Check sheet for the modelled part. Datum: model origin and axes. Units: mm. Round coordinates to 2 decimals unless told otherwise and drop trailing zeros. Write each loop counter-clockwise with the first axis right and the second up, starting at its lowest first coordinate (ties: lowest second). Pieces come first, ordered by that corner, then holes. Notation, with made-up numbers: (2.5, -28) - (8.5, -28) arc R34 cw to (8.5, 11) - close; hole circle Ø5 at (68, 20). An arc over 180 degrees is marked (long way). Answer as a JSON object with one key per item and string values. Group by question number.
Item 1: Sectioned sample at A-A on x = 90.5. Record the boundary of the cut face in (y, z) (3 decimals), plus the area to 3 significant figures.
Item 2: Thickness scan on line 1 (Y direction, x = 118.11, z = 1) (3 decimals); line 2 (Y direction, x = -101.6, z = 0.75); line 3 (Y direction, x = 139, z = 2.95). Record the ranges inside material, lowest first.
Item 3: Gauge pin test, flat ends, axial feed: P1, Ø5, axis at x = 139.7, y = 0, coming from the -Z side; P2, Ø8, axis at x = -101.6, y = 97.79, coming from the +Z side (3 decimals). Record the tip position at first contact, or that the pin passes through.
Item 4: Sectioned sample at B-B on z = 1.45. Count the separate pieces of the cut face and the enclosed holes in it, plus the area to 3 significant figures.
```python
from build123d import *

# Parameters (mm, degrees)
SKETCH1_W           = 304.8
SKETCH1_H           = 304.8
SKETCH1_R           = 2.54
SKETCH1_R_2         = 3.2639
BOSS_EXTRUDE1_DEPTH = 3.175


with BuildPart() as part:
    # Sketch1 → Boss-Extrude1 (new body)
    with BuildSketch(Plane.XY):
        Rectangle(SKETCH1_W, SKETCH1_H)
        with Locations((-50.8, 127)):
            Circle(SKETCH1_R, mode=Mode.SUBTRACT)
        with Locations((0, 127)):
            Circle(SKETCH1_R, mode=Mode.SUBTRACT)
        with Locations((50.8, 127)):
            Circle(SKETCH1_R, mode=Mode.SUBTRACT)
        with Locations((50.8, -127)):
            Circle(SKETCH1_R, mode=Mode.SUBTRACT)
        with Locations((0, -127)):
            Circle(SKETCH1_R, mode=Mode.SUBTRACT)
        with Locations((-50.8, -127)):
            Circle(SKETCH1_R, mode=Mode.SUBTRACT)
        with Locations((-101.6, 97.79)):
            Circle(SKETCH1_R, mode=Mode.SUBTRACT)
        with Locations((0, 97.79)):
            Circle(SKETCH1_R, mode=Mode.SUBTRACT)
        with Locations((101.6, 97.79)):
            Circle(SKETCH1_R, mode=Mode.SUBTRACT)
        with Locations((101.6, 127)):
            Circle(SKETCH1_R, mode=Mode.SUBTRACT)
        with Locations((-101.6, 127)):
            Circle(SKETCH1_R, mode=Mode.SUBTRACT)
        with Locations((-118.11, 33.02)):
            Circle(SKETCH1_R, mode=Mode.SUBTRACT)
        with Locations((-101.6, -127)):
            Circle(SKETCH1_R, mode=Mode.SUBTRACT)
        with Locations((101.6, -127)):
            Circle(SKETCH1_R, mode=Mode.SUBTRACT)
        with Locations((101.6, -97.79)):
            Circle(SKETCH1_R, mode=Mode.SUBTRACT)
        with Locations((0, -97.79)):
            Circle(SKETCH1_R, mode=Mode.SUBTRACT)
        with Locations((-101.6, -97.79)):
            Circle(SKETCH1_R, mode=Mode.SUBTRACT)
        with Locations((-118.11, -33.02)):
            Circle(SKETCH1_R, mode=Mode.SUBTRACT)
        with Locations((-139.7, 139.7)):
            Circle(SKETCH1_R_2, mode=Mode.SUBTRACT)
        with Locations((-139.7, 0)):
            Circle(SKETCH1_R_2, mode=Mode.SUBTRACT)
        with Locations((-139.7, -139.7)):
            Circle(SKETCH1_R_2, mode=Mode.SUBTRACT)
        with Locations((139.7, -139.7)):
            Circle(SKETCH1_R_2, mode=Mode.SUBTRACT)
        with Locations((139.7, 0)):
            Circle(SKETCH1_R_2, mode=Mode.SUBTRACT)
        with Locations((139.7, 139.7)):
            Circle(SKETCH1_R_2, mode=Mode.SUBTRACT)
        with Locations((118.11, -33.02)):
            Circle(SKETCH1_R, mode=Mode.SUBTRACT)
        with Locations((118.11, 33.02)):
            Circle(SKETCH1_R, mode=Mode.SUBTRACT)
        with BuildLine():
            Line((-101.6, 78.74), (101.6, 78.74))
            ThreePointArc((101.6, 78.74), (106.090128061, 76.880128061), (107.95, 72.39))
            Line((107.95, 72.39), (107.95, 24.765))
            ThreePointArc((107.95, 24.765), (108.693948776, 22.968948776), (110.49, 22.225))
            Line((110.49, 22.225), (120.65, 22.225))
            ThreePointArc((120.65, 22.225), (125.140128061, 20.365128061), (127, 15.875))
            Line((127, 15.875), (127, -15.875))
            ThreePointArc((127, -15.875), (125.140128061, -20.365128061), (120.65, -22.225))
            Line((120.65, -22.225), (110.49, -22.225))
            ThreePointArc((110.49, -22.225), (108.693948776, -22.968948776), (107.95, -24.765))
            Line((107.95, -24.765), (107.95, -72.39))
            ThreePointArc((107.95, -72.39), (106.090128061, -76.880128061), (101.6, -78.74))
            Line((101.6, -78.74), (-101.6, -78.74))
            ThreePointArc((-101.6, -78.74), (-106.090128061, -76.880128061), (-107.95, -72.39))
            Line((-107.95, -72.39), (-107.95, -24.765))
            ThreePointArc((-107.95, -24.765), (-108.693948776, -22.968948776), (-110.49, -22.225))
            Line((-110.49, -22.225), (-120.65, -22.225))
            ThreePointArc((-120.65, -22.225), (-125.140128061, -20.365128061), (-127, -15.875))
            Line((-127, -15.875), (-127, 15.875))
            ThreePointArc((-127, 15.875), (-125.140128061, 20.365128061), (-120.65, 22.225))
            Line((-120.65, 22.225), (-110.49, 22.225))
            ThreePointArc((-110.49, 22.225), (-108.693948776, 22.968948776), (-107.95, 24.765))
            Line((-107.95, 24.765), (-107.95, 72.39))
            ThreePointArc((-107.95, 72.39), (-106.090128061, 76.880128061), (-101.6, 78.74))
        make_face(mode=Mode.SUBTRACT)
    extrude(amount=BOSS_EXTRUDE1_DEPTH)


solid = part.part
```
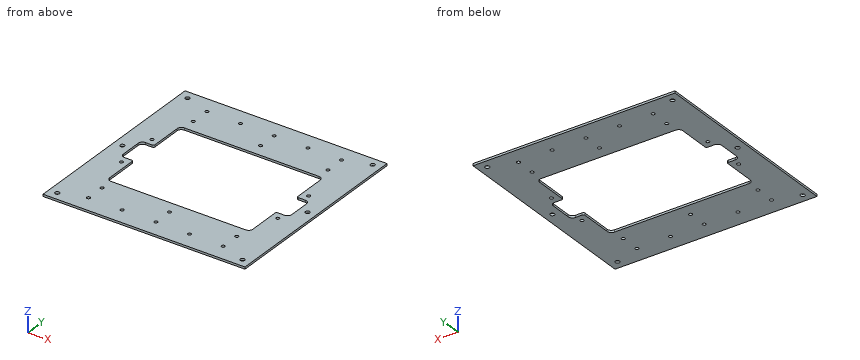
Completed:
{
 "1": {"outline": "(-152.4, 0) - (-78.74, 0) - (-78.74, 3.175) - (-152.4, 3.175) - close; (78.74, 0) - (152.4, 0) - (152.4, 3.175) - (78.74, 3.175) - close", "area": "468 mm²"},
 "2": {"line 1": "-152.4 to -35.56, -30.48 to -22.225, 22.225 to 30.48, 35.56 to 152.4", "line 2": "-152.4 to -129.54, -124.46 to -100.33, -95.25 to -78.74, 78.74 to 95.25, 100.33 to 124.46, 129.54 to 152.4", "line 3": "-152.4 to -142.89, -136.51 to -3.19, 3.19 to 136.51, 142.89 to 152.4"},
 "3": {"P1": "through", "P2": "z = 3.175"},
 "4": {"separate pieces": "1", "enclosed holes": "27", "area": "56,700 mm²"}
}
